Check sheet for the modelled part. Datum: model origin and axes. Units: mm. Face numbers are marked on the shaded views. A direction names the side the tool comes from. Round coordinates to 2 decimals unless told otherwise and drop trailing zeros. Write each loop counter-clockwise with the first axis right and the second up, starting at its lowest first coordinate (ties: lowest second). Pieces come first, ordered by that corner, then holes. Notation, with made-up numbers: M -34.75,64.25 L 9.25,64.25 A15 ccw 9.25,73.25 Z; hole C 43,-24.75 d3. An arc over 180 degrees is marked long. Answer in a Markdown table with one row per item.
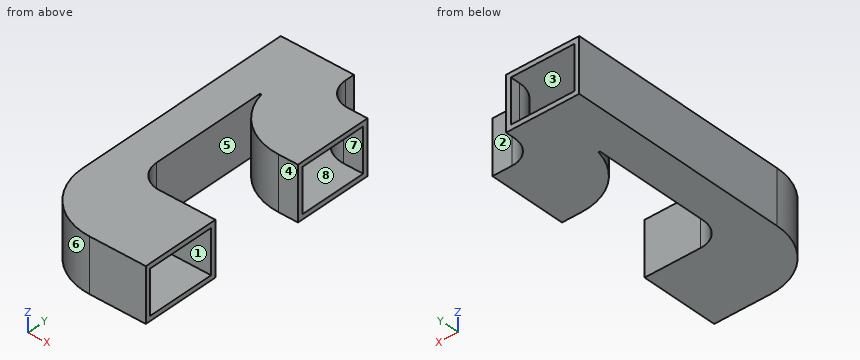
```python
from build123d import *

# Parameters (mm, degrees)
RESSALTO_EXTRUS_O1_DEPTH = 11
CASCA2_T                 = -1


with BuildPart() as part:
    # Esboço1 → Ressalto-extrusão1 (new body)
    with BuildSketch(Plane.XY):
        with BuildLine():
            Line((0, 45.5), (0, 0))
            ThreePointArc((0, 0), (3.661165235, -8.838834765), (12.5, -12.5))
            Line((12.5, -12.5), (24, -12.5))
            Line((24, -12.5), (24, 3.5))
            Line((24, 3.5), (12.5, 3.5))
            ThreePointArc((12.5, 3.5), (8.964466094, 4.964466094), (7.5, 8.5))
            Line((7.5, 8.5), (7.5, 32.277868482))
            Line((7.5, 32.277868482), (7.8, 32.277868482))
            ThreePointArc((7.8, 32.277868482), (12.182604141, 25.246112468), (20, 22.5))
            Line((20, 22.5), (24, 22.5))
            Line((24, 22.5), (24, 38.5))
            Line((24, 38.5), (20, 38.5))
            ThreePointArc((20, 38.5), (16.464466094, 39.964466094), (15, 43.5))
            Line((15, 43.5), (15, 45.5))
            Line((15, 45.5), (0, 45.5))
        make_face()
    extrude(amount=RESSALTO_EXTRUS_O1_DEPTH)

    # Casca2
    casca2_openings = [part.faces().sort_by_distance(p)[0] for p in [
        (24, 30.5, 5.5),
        (24, -4.5, 5.5),
        (7.5, 45.5, 5.5),
    ]]
    offset(amount=CASCA2_T, openings=casca2_openings, kind=Kind.INTERSECTION)


solid = part.part
```
1. Section check D-D, the plane y = 20. Record the cut outline in (x, z).
Found:
| item | result |
|---|---|
| outline | M 0,0 L 7.5,0 L 7.5,11 L 0,11 Z; hole M 1,1 L 6.5,1 L 6.5,10 L 1,10 Z |
2. Go/stop test with flat-tipped pins: pin 1 (6 mm diameter, centred on x = 20.5, z = 1.5, fed in from +Y); pin 2 (2 mm diameter, centred on x = 8.5, z = 2, fed in from -Y); pin 3 (2 mm diameter, centred on x = 10, z = 9, fed in from -Y). Record where each tip stops, or that it passes through.
Found:
| item | result |
|---|---|
| pin 1 | stops at y = 39.17 |
| pin 2 | stops at y = -12.13 |
| pin 3 | stops at y = -12.41 |
3. Draft check along X on the marked faces 6, 7 and 8. Enter one of: +X half, -X half, draft (parallel to the pull), parting line (faces both ways), or undercut.
Found:
| item | result |
|---|---|
| face 6 | -X half |
| face 7 | draft |
| face 8 | undercut |
4. Section check C-C, the plane x = 11.5. Record the cut outline in (y, z).
Found:
| item | result |
|---|---|
| outline | M -12.46,0 L 3.6,0 L 3.6,11 L -12.46,11 Z; M 25.83,0 L 45.5,0 L 45.5,1 L 27.25,1 L 27.25,10 L 45.5,10 L 45.5,11 L 25.83,11 Z; hole M -11.46,1 L 2.58,1 L 2.58,10 L -11.46,10 Z |
5. Access from +Z, -Z, +X, -X, +Y, -Y to the whole of each face (thin tool, end or side, straight path). Record for the marked faces 1, 2, 3, 4 and 5.
Found:
| item | result |
|---|---|
| face 1 | +X |
| face 2 | +Z, -Z, +X, +Y |
| face 3 | none |
| face 4 | +Z, -Z, +X |
| face 5 | +Z, -Z |
6. Scan lines: L1, parallel to Y at x = 20, z = 3; L2, parallel to X at y = 9.5, z = 3; L3, parallel to Z at x = 11.75, y = -6. Record each from-to range of solid material in increasing order.
Found:
| item | result |
|---|---|
| L1 | y = -12.5 to -11.5, 2.5 to 3.5, 22.5 to 23.5, 37.5 to 38.5 |
| L2 | x = 0 to 1, 6.5 to 7.5 |
| L3 | z = 0 to 1, 10 to 11 |
7. Section check A-A, the plane z = 4.25. Count the separate pieces of the cut face and the enclosed holes in it, and give its area (3 significant figures).
Found:
| item | result |
|---|---|
| separate pieces | 3 |
| enclosed holes | 0 |
| area | 157 mm2 |
8. Section check B-B, the plane x = 20.75. Record the cut outline in (y, z), and give its area (4 significant figures).
Found:
| item | result |
|---|---|
| outline | M -12.5,0 L 3.5,0 L 3.5,11 L -12.5,11 Z; M 22.5,0 L 38.5,0 L 38.5,11 L 22.5,11 Z; hole M -11.5,1 L 2.5,1 L 2.5,10 L -11.5,10 Z; hole M 23.5,1 L 37.5,1 L 37.5,10 L 23.5,10 Z |
| area | 100.0 mm2 |
